Job drawing, mm, ordinate dimensions from the low corner. One solid piece. A direction names the side the tool comes from. Coordinates: 2 decimals unless noted, no trailing zeros. Loops run counter-clockwise (first coordinate to the right, second up) from the corner with the lowest first, then second, coordinate; pieces in that order, holes last. Notation, with made-up numbers: M 15.5,-2 L 58.5,-2 A11 cw 58.5,13 Z; hole C 61,-16 d10. An arc over 180 degrees is marked long. Answer as a JSON object with one key per item and string values. Group by question number.
1. Mould opens along X. For the marked faces 1, 2 and 3 say: released by +X, released by -X, zero draft, split by the parting line, or undercut.
2. Saw through at C-C on y = 10. Write the cut outline in (x, z), then the cut area to 3 significant figures.
3. Saw through at B-B on z = 17. Write the cut outline in (x, y).
4. Saw through at A-A on x = 36. Write the cut outline in (y, z).
5. 3-axis set-ups, long thin cutter, end or side, ignore diameter. For the marked faces 4, 5, 6, 7 and 8: which of +Z, -Z, +X, -X, +Y, -Y reach the whole face in a straight line?
6. Saw through at D-D on y = 2. Write the cut outline in (x, z), then the cut area to 3 significant figures.
7. Drill centre lines: L1, parallel to X at y = 14, z = 10.75; L2, parallel to Y at x = 4, z = 26.3; L3, parallel to X at y = 13.5, z = 24.5. Where is each one in solid material? Low to high.
8. Drop flat-ended pins along their axis: pin 1 Ø6 at (y, z) = (8.5, 16) entering from -X; pin 2 Ø1 at (y, z) = (9, 12) entering from +X; pin 3 Ø3 at (x, y) = (43, 13.5) entering from +Z. Give the stop position or say it passes through.
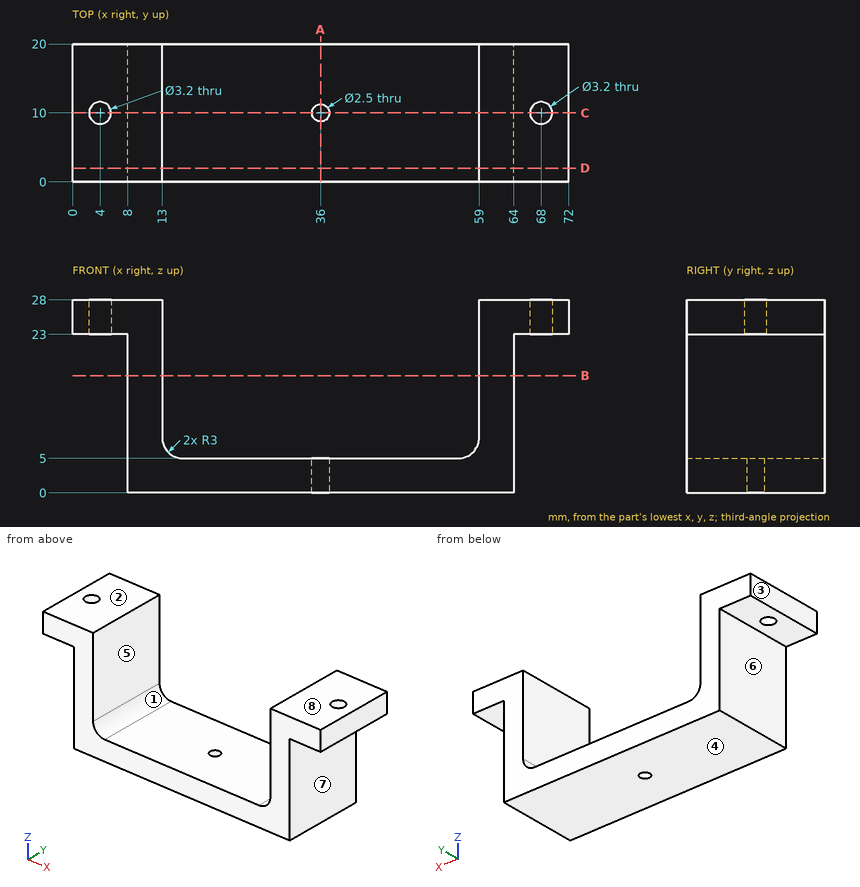
Outcome:
{
 "1": {"face 1": "undercut", "face 2": "zero draft", "face 3": "released by -X"},
 "2": {"outline": "M 0,23 L 2.4,23 L 2.4,28 L 0,28 Z; M 5.6,23 L 8,23 L 8,0 L 34.75,0 L 34.75,5 L 16,5 A3 cw 13,8 L 13,28 L 5.6,28 Z; M 37.25,0 L 64,0 L 64,23 L 66.4,23 L 66.4,28 L 59,28 L 59,8 A3 cw 56,5 L 37.25,5 Z; M 69.6,23 L 72,23 L 72,28 L 69.6,28 Z", "area": "549 mm²"},
 "3": {"outline": "M 8,0 L 13,0 L 13,20 L 8,20 Z; M 59,0 L 64,0 L 64,20 L 59,20 Z"},
 "4": {"outline": "M 0,0 L 8.75,0 L 8.75,5 L 0,5 Z; M 11.25,0 L 20,0 L 20,5 L 11.25,5 Z"},
 "5": {"face 4": "-Z, +X, -X, +Y, -Y", "face 5": "+Z, +Y, -Y", "face 6": "-Z, -X, +Y, -Y", "face 7": "-Z, +X, +Y, -Y", "face 8": "+Z, +X, -X, +Y, -Y"},
 "6": {"outline": "M 0,23 L 8,23 L 8,0 L 64,0 L 64,23 L 72,23 L 72,28 L 59,28 L 59,8 A3 cw 56,5 L 16,5 A3 cw 13,8 L 13,28 L 0,28 Z", "area": "594 mm²"},
 "7": {"L1": "x = 8 to 13, 59 to 64", "L2": "y = 0 to 8.4, 11.6 to 20", "L3": "x = 0 to 13, 59 to 72"},
 "8": {"pin 1": "stops at x = 8", "pin 2": "stops at x = 64", "pin 3": "stops at z = 5"}
}
